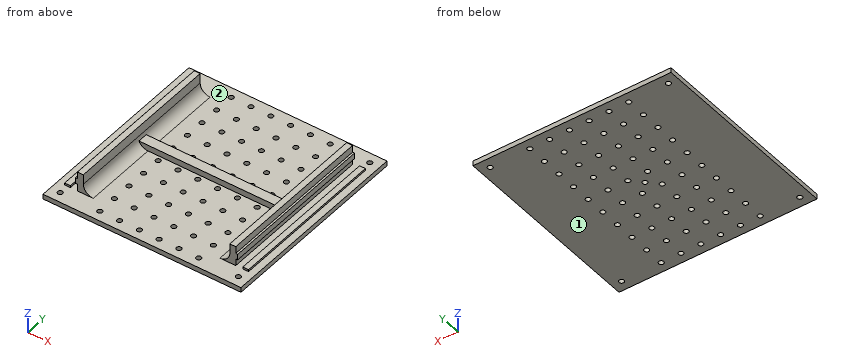
```python
from build123d import *

# Parameters (mm, degrees)
SKETCH1_W            = 100
SKETCH1_H            = 100
MAIN_DEPTH           = 12.5
CUT_EXTRUDE1_DEPTH   = 51
SKETCH3_W            = 74
SKETCH3_H            = 10
CUT_EXTRUDE2_DEPTH   = 101
FILLET1_R            = 5
SKETCH9_W            = 80
SKETCH9_H            = 5
BOSS_EXTRUDE1_DEPTH  = 3
SKETCH4_R            = 1.25
FIXHOLE_DEPTH        = 3.5
LPATTERN1_COUNT      = 6
LPATTERN1_PITCH      = 10
LPATTERN1_COUNT_DIR2 = 10
LPATTERN1_PITCH_DIR2 = 10
SKETCH6_R            = 1.25
CENTRALHOLE_DEPTH    = 3.5
SKETCH7_W            = 100
SKETCH7_H            = 10
CUT_EXTRUDE3_DEPTH   = 10
SKETCH8_R            = 1.25
CUT_EXTRUDE4_DEPTH   = 3.5
LPATTERN2_COUNT      = 2
LPATTERN2_PITCH      = 90
LPATTERN2_COUNT_DIR2 = 2
LPATTERN2_PITCH_DIR2 = 90


with BuildPart() as part:
    # Sketch1 → Main (new body)
    with BuildSketch(Plane.XY):
        Rectangle(SKETCH1_W, SKETCH1_H)
    extrude(amount=MAIN_DEPTH)

    # Sketch2 → Cut-Extrude1 (cut, symmetric)
    with BuildSketch(Plane(origin=(0, 0, 0), x_dir=(1, 0, 0), z_dir=(0, 1, 0))):
        Polygon((-40, -8.95), (-40, -12.5), (-50, -12.5), (-50, -2.5), (-46.45, -2.5), (-46.45, -3.5), (-43.55, -3.5), (-43.55, -2.5), (-40, -2.5), (-40, -6.05), (-41, -6.05), (-41, -8.95), align=None)
    cut_extrude1 = extrude(amount=CUT_EXTRUDE1_DEPTH, both=True, mode=Mode.SUBTRACT)

    # Mirror1: Cut-Extrude1 across plane
    add(cut_extrude1.mirror(Plane(origin=(0, 0, 0), x_dir=(0, 0, 1), z_dir=(1, 0, 0))), mode=Mode.SUBTRACT)

    # Sketch3 → Cut-Extrude2 (cut, through all)
    with BuildSketch(Plane(origin=(0, 50, 0), x_dir=(1, 0, 0), z_dir=(0, 1, 0))):
        with Locations((0, -7.5)):
            Rectangle(SKETCH3_W, SKETCH3_H)
    extrude(amount=-CUT_EXTRUDE2_DEPTH, mode=Mode.SUBTRACT)

    # Fillet1
    fillet1_edges = [part.edges().sort_by_distance(p)[0] for p in [
        (-37, 0, 2.5),
        (37, 0, 2.5),
    ]]
    fillet(fillet1_edges, radius=FILLET1_R)

    # Sketch9 → Boss-Extrude1 (add)
    with BuildSketch(Plane.XY.offset(2.5)):
        Rectangle(SKETCH9_W, SKETCH9_H)
    extrude(amount=BOSS_EXTRUDE1_DEPTH)

    # Sketch4 → FixHole (cut, through all)
    with BuildSketch(Plane.XY.offset(2.5)):
        with Locations((25, -45)):
            Circle(SKETCH4_R)
    fixhole = extrude(amount=-FIXHOLE_DEPTH, mode=Mode.SUBTRACT)

    # LPattern1: FixHole 6 × 10
    with Locations(*[(-i * LPATTERN1_PITCH, j * LPATTERN1_PITCH_DIR2, 0) for i in range(LPATTERN1_COUNT) for j in range(LPATTERN1_COUNT_DIR2) if (i, j) != (0, 0)]):
        add(fixhole, mode=Mode.SUBTRACT)

    # Sketch6 → CentralHole (cut, through all)
    with BuildSketch(Plane.XY.offset(2.5)):
        Circle(SKETCH6_R)
    extrude(amount=-CENTRALHOLE_DEPTH, mode=Mode.SUBTRACT)

    # Sketch7 → Cut-Extrude3 (cut)
    with BuildSketch(Plane(origin=(0, 0, 12.5), x_dir=(-1, 0, 0), z_dir=(0, 0, -1))):
        with Locations((0, -45)):
            Rectangle(SKETCH7_W, SKETCH7_H)
        with Locations((0, 45)):
            Rectangle(SKETCH7_W, SKETCH7_H)
    extrude(amount=CUT_EXTRUDE3_DEPTH, mode=Mode.SUBTRACT)

    # Sketch8 → Cut-Extrude4 (cut, through all)
    with BuildSketch(Plane.XY.offset(2.5)):
        with Locations((-45, 45)):
            Circle(SKETCH8_R)
    cut_extrude4 = extrude(amount=-CUT_EXTRUDE4_DEPTH, mode=Mode.SUBTRACT)

    # LPattern2: Cut-Extrude4 2 × 2
    with Locations(*[(i * LPATTERN2_PITCH, -j * LPATTERN2_PITCH_DIR2, 0) for i in range(LPATTERN2_COUNT) for j in range(LPATTERN2_COUNT_DIR2) if (i, j) != (0, 0)]):
        add(cut_extrude4, mode=Mode.SUBTRACT)


solid = part.part
```
Design review of the part built by this model. Coordinates are the model's own, in mm. Face numbers are marked on the shaded views. Coordinates: 2 decimals unless noted, no trailing zeros. Order: outer loops, then holes, each group sorted by start corner. A loop starts at its lowest first (then second) coordinate and runs counter-clockwise, first axis right, second up. Notation, with made-up numbers: (2, -17) - (47, -17) arc R37 cw to (47, 19) - close; hole circle Ø2 at (46, 21). An arc over 180 degrees is marked (long way). One line per question, with ' | ' between items.
Q1. Consider section A-A, the plane x = 45. Give the boundary of the cut face in (y, z).
Answer key:
outline: (-50, 0) - (-46.25, 0) - (-46.25, 2.5) - (-50, 2.5) - close; (-43.75, 0) - (43.75, 0) - (43.75, 2.5) - (40, 2.5) - (40, 3.5) - (-40, 3.5) - (-40, 2.5) - (-43.75, 2.5) - close; (46.25, 0) - (50, 0) - (50, 2.5) - (46.25, 2.5) - close
Q2. Consider section C-C, the plane x = -20. Give the boundary of the cut face in (y, z), then the cut area to 3 significant figures.
Answer key:
outline: (-50, 0) - (50, 0) - (50, 2.5) - (2.5, 2.5) - (2.5, 5.5) - (-2.5, 5.5) - (-2.5, 2.5) - (-50, 2.5) - close | area: 265 mm2
Q3. The part is to be moulded in two halves that separate along X. For the marked faces 1 and 2, say which applies: +X half, -X half, draft (parallel to the pull), parting line (faces both ways), or undercut.
Answer key:
face 1: draft | face 2: undercut
Q4. Clearance check with flat-ended pins moving along their axes: pin 1 Ø3 at (x, y) = (24, 38.5) entering from +Z; pin 2 Ø5 at (y, z) = (36, 8) entering from -X; pin 3 Ø1.1 at (y, z) = (18, 4.5) entering from -X; pin 4 Ø3 at (x, y) = (15, -15) entering from -Z. State where each tip first meets the part, or that it passes through.
Answer key:
pin 1: stops at z = 2.5 | pin 2: stops at x = -41 | pin 3: stops at x = -40 | pin 4: stops at z = 0
Q5. To check wall thickness, follow line 1 along X through (y, z) = (-21, 11); line 2 along Z through (x, y) = (-11.5, -37.5); line 3 along Z through (x, y) = (6.5, 0.5). State the ranges of each line that lie inside material, in increasing order.
Answer key:
line 1: x = -40 to -37, 37 to 40 | line 2: z = 0 to 2.5 | line 3: z = 0 to 5.5
Q6. Consider section D-D, the plane y = -45. Give the number of separate pieces and of enclosed holes in the cut face, then the cut area to 3 significant figures.
Answer key:
separate pieces: 9 | enclosed holes: 0 | area: 200 mm2
